The listing builds one solid part. Answer for the finished solid, in the listing's coordinates (mm). A direction names the side the tool comes from. Round coordinates to 2 decimals unless told otherwise and drop trailing zeros. Loops run counter-clockwise (first coordinate to the right, second up) from the corner with the lowest first, then second, coordinate; pieces in that order, holes last. Notation, with made-up numbers: (2.25, 68) -> (39.25, 68) arc R26 ccw to (39.25, 101) -> close; hole circle Ø9 at (9.5, 71). An arc over 180 degrees is marked (long way). Use a Markdown table: item, result. Add a question column.
Q1. Section A-A on y = 0 is taken. Give the vertices of the cut face in (x, z), then the cut area to 3 significant figures.
Q2. For a pull along Z with two mould halves and no side action, classify faces 1 (the flat face through (4, 0, 20)), 2 (the flat face through (0, 0, 40)), 3 (the flat face through (-4.76, -0.06, 26.44)), 4 (the cylindrical face through (2.769, -5.323, 19.72)) as released by +Z, released by -Z, zero draft, split by the parting line, or undercut.
Q3. Section C-C on z = 17.5 is taken. Give the vertices of the cut face in (x, y), then the cut area to 3 significant figures.
Q4. Consider line 1 (X direction, y = -2.5, z = 22); line 2 (Y direction, x = 4, z = 28); line 3 (Y direction, x = 1.75, z = 12.5). Determine where each line is inside the solid, lowest interval first.
Q5. Section D-D on x = 2 is taken. Give the vertices of the cut face in (y, z).
Q6. Which of the six approach directions +Z, -Z, +X, -X, +Y, -Y give full straight-line access (tool end or side, diameter ignored) to faces 5 (the flat face through (5, 0, 26)), 6 (the flat face through (0, 0, 0)), 7 (the flat face through (-4, 0, 20))?
Q7. Section B-B on x = 4.75 is taken. Give the vertices of the cut face in (y, z), then the cut area to 3 significant figures.
Q8. Given pin 1 Ø1 at (x, z) = (-5, 5.5) entering from -Y; pin 2 Ø1.5 at (x, z) = (4.5, 18) entering from -Y; pin 3 Ø2.5 at (y, z) = (-1.5, 19) entering from +X, each flat-ended and moving along its own axis, determine where each tip first touches the part or whether it passes through.
from build123d import *

# Parameters (mm, degrees)
SKETCH_1_R          = 6
EXTRUDE_1_DEPTH     = 40
SKETCH_3_W          = 12
SKETCH_3_H          = 9
CUT_EXTRUDE_1_DEPTH = 40
DRAFT_3_ANGLE       = 30


with BuildPart() as part:
    # 草图1 → 凸台-拉伸1 (new body)
    with BuildSketch(Plane.XY):
        Circle(SKETCH_1_R)
    extrude(amount=EXTRUDE_1_DEPTH)

    # 草图3 → 切除-拉伸1 (cut)
    with BuildSketch(Plane(origin=(4, 0, 0), x_dir=(0, 0, -1), z_dir=(1, 0, 0))):
        with Locations((-20, 0)):
            Rectangle(SKETCH_3_W, SKETCH_3_H)
    cut_extrude_1 = extrude(amount=CUT_EXTRUDE_1_DEPTH, mode=Mode.SUBTRACT)

    # 镜向1: 切除-拉伸1 across plane
    add(cut_extrude_1.mirror(Plane(origin=(0, 0, 0), x_dir=(0, 0, 1), z_dir=(1, 0, 0))), mode=Mode.SUBTRACT)

    # 拔模3
    draft_3_faces = [part.faces().sort_by_distance(p)[0] for p in [
        (-4.812657334, 0, 26),
    ]]
    draft(draft_3_faces, Plane(origin=(-4, 0, 0), x_dir=(0, 0, -1), z_dir=(-1, 0, 0)), DRAFT_3_ANGLE)


solid = part.part
Checked values:
| question | item | result |
|---|---|---|
| 1 | outline | (-6, 0) -> (6, 0) -> (6, 14) -> (4, 14) -> (4, 26) -> (6, 26) -> (6, 40) -> (-6, 40) -> (-6, 27.15) -> (-4, 26) -> (-4, 14) -> (-6, 14) -> close |
| 1 | area | 431 mm2 |
| 2 | face 1 | undercut |
| 2 | face 2 | released by +Z |
| 2 | face 3 | undercut |
| 2 | face 4 | zero draft |
| 3 | outline | (-4, -4.47) arc R6 ccw to (4, -4.47) -> (4, 4.47) arc R6 ccw to (-4, 4.47) -> close |
| 3 | area | 88.3 mm2 |
| 4 | line 1 | x = -4 to 4 |
| 4 | line 2 | y = -4.47 to 4.47 |
| 4 | line 3 | y = -5.74 to 5.74 |
| 5 | outline | (-5.66, 0) -> (5.66, 0) -> (5.66, 40) -> (-5.66, 40) -> close |
| 6 | face 5 | +X, +Y, -Y |
| 6 | face 6 | -Z, +X, -X, +Y, -Y |
| 6 | face 7 | -X, +Y, -Y |
| 7 | outline | (-3.67, 0) -> (3.67, 0) -> (3.67, 14) -> (-3.67, 14) -> close; (-3.67, 26) -> (3.67, 26) -> (3.67, 40) -> (-3.67, 40) -> close |
| 7 | area | 205 mm2 |
| 8 | pin 1 | stops at y = -3.97 |
| 8 | pin 2 | stops at y = -4.68 |
| 8 | pin 3 | stops at x = 4 |
